```python
from build123d import *

# Parameters (mm, degrees)
PAD_DEPTH = 5


with BuildPart() as part:
    # Sketch → Pad (new body, symmetric)
    with BuildSketch(Plane.YZ):
        with BuildLine():
            ThreePointArc((-22.5, 25), (-24.267767, 24.267767), (-25, 22.5))
            Line((-25, -22.5), (-25, 22.5))
            ThreePointArc((-25, -22.5), (-24.267767, -24.267767), (-22.5, -25))
            Line((22.5, -25), (-22.5, -25))
            ThreePointArc((22.5, -25), (24.267767, -24.267767), (25, -22.5))
            Line((25, 22.5), (25, -22.5))
            ThreePointArc((25, 22.5), (24.267767, 24.267767), (22.5, 25))
            Line((-22.5, 25), (22.5, 25))
        make_face()
        with BuildLine():
            ThreePointArc((-22.5, 24), (-23.56066, 23.56066), (-24, 22.5))
            Line((-24, -22.5), (-24, 22.5))
            ThreePointArc((-24, -22.5), (-23.56066, -23.56066), (-22.5, -24))
            Line((22.5, -24), (-22.5, -24))
            ThreePointArc((22.5, -24), (23.56066, -23.56066), (24, -22.5))
            Line((24, 22.5), (24, -22.5))
            ThreePointArc((24, 22.5), (23.56066, 23.56066), (22.5, 24))
            Line((-22.5, 24), (22.5, 24))
        make_face(mode=Mode.SUBTRACT)
    extrude(amount=PAD_DEPTH, both=True)


solid = part.part
```
Here's how the part is built. I have some questions about the finished solid (model axes, mm). A direction names the side the tool comes from. Give positions to 0.01 mm unless a question says otherwise; leave off trailing zeros. Order: outer loops, then holes, each group sorted by start corner. A loop starts at its lowest first (then second) coordinate and runs counter-clockwise, first axis right, second up. Notation, with made-up numbers: (3, 59) -> (27, 59) arc R27 ccw to (27, 98) -> close; hole circle Ø4 at (-33.5, 50). An arc over 180 degrees is marked (long way). Use CSV: the item, a comma, the result in double quotes. Start each with the question number.
Item 1: Suppose I cut it at A-A (x = -1.25). List the corners of the cut face in (y, z) for me, and give its area (3 significant figures).
Item 2: I'm going to push a flat-ended pin straight in: P1, Ø12, axis at y = -16.5, z = -0.5, coming from the +X side. Where does the tip first touch, or does it pass through?
Item 3: If I drill on probe 1 along Z at (x, y) = (-4, 17), over which ranges is the centre line in solid material (lowest first)? Write a range as [from, to].
Item 4: On a 3-axis mill with a long thin cutter (end or side, diameter ignored), from which of +Z, -Z, +X, -X, +Y, -Y can I reach the whole of each face in a straight line? I mean faces 1 (the cylindrical face through (0.07, 24.287, 24.248)), 2 (the flat face through (0, 0, 24)). Say none if no direction works.
Item 5: Thinking about a two-plate mould opening in Y: for faces 3 (the flat face through (0, 24, 0)), 4 (the cylindrical face through (0.07, -24.248, 24.287)), 5 (the flat face through (-5, -11.2, 24.2)), 6 (the flat face through (0, 25, 0)), which applies, pulls with the +Y half, pulls with the -Y half, needs draft (parallel to the pull), parting line crosses it, or undercut?
Item 6: Suppose I cut it at B-B (y = 16). List the corners of the cut face in (x, z) for me, and give its area (3 significant figures).
Answer block:
1,outline,"(-25, -22.5) arc R2.5 ccw to (-22.5, -25) -> (22.5, -25) arc R2.5 ccw to (25, -22.5) -> (25, 22.5) arc R2.5 ccw to (22.5, 25) -> (-22.5, 25) arc R2.5 ccw to (-25, 22.5) -> close; hole (-24, -22.5) arc R1.5 ccw to (-22.5, -24) -> (22.5, -24) arc R1.5 ccw to (24, -22.5) -> (24, 22.5) arc R1.5 ccw to (22.5, 24) -> (-22.5, 24) arc R1.5 ccw to (-24, 22.5) -> close"
1,area,"193 mm^2"
2,P1,"passes through"
3,probe 1,"z = [-25, -24], [24, 25]"
4,face 1,"+Z, +X, -X, +Y"
4,face 2,"+X, -X"
5,face 3,"undercut"
5,face 4,"pulls with the -Y half"
5,face 5,"needs draft"
5,face 6,"pulls with the +Y half"
6,outline,"(-5, -25) -> (5, -25) -> (5, -24) -> (-5, -24) -> close; (-5, 24) -> (5, 24) -> (5, 25) -> (-5, 25) -> close"
6,area,"20.0 mm^2"
